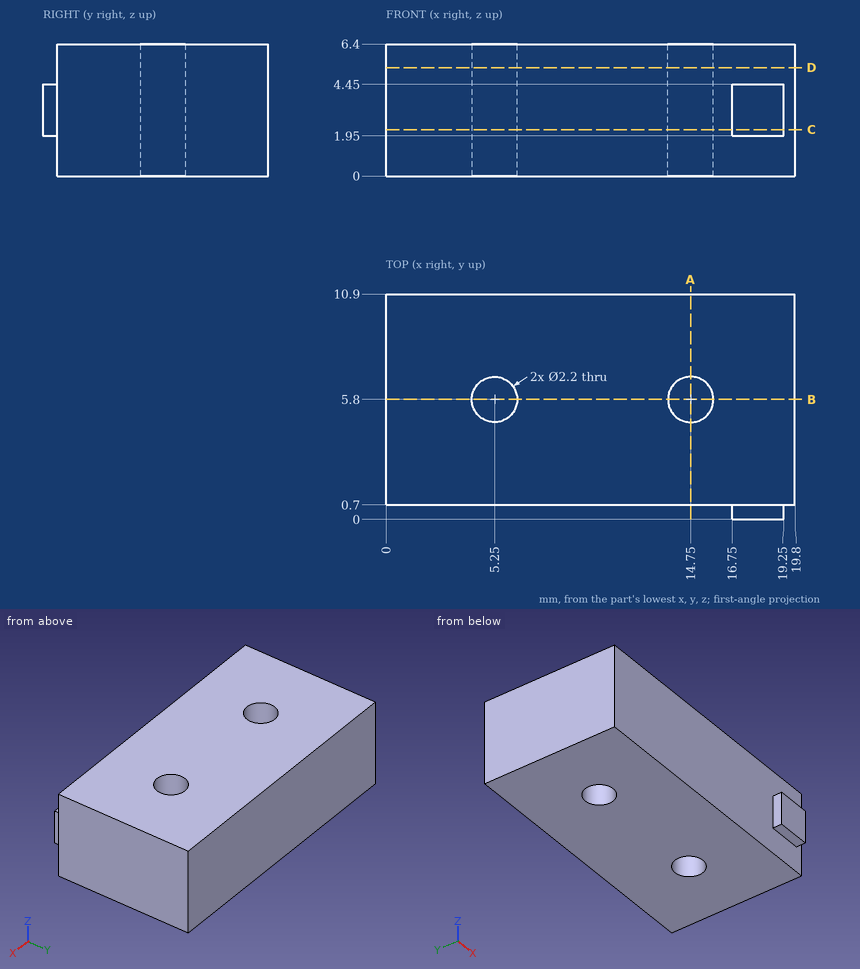
Can you work these out from the drawing? Everything is in mm from the part's minimum corner. Round coordinates to 2 decimals unless told otherwise and drop trailing zeros. Write each loop counter-clockwise with the first axis right and the second up, starting at its lowest first coordinate (ties: lowest second). Pieces come first, ordered by that corner, then holes.
1. Suppose I cut it at D-D (z = 5.25). List the corners of the cut face in (x, y) for me, and give its area (3 significant figures).
2. Suppose I cut it at A-A (x = 14.75). List the corners of the cut face in (y, z) for me.
3. Suppose I cut it at B-B (y = 5.8). List the corners of the cut face in (x, z) for me.
4. I need wall thicknesses on L1, parallel to X at y = 5.8, z = 4; L2, parallel to Y at x = 14.75, z = 2.5; L3, parallel to Y at x = 8.5, z = 1.25. Which ranges of each line are inside material? Lowest first, please.
5. Suppose I cut it at C-C (z = 2.25). List the corners of the cut face in (x, y) for me, and give its area (3 significant figures).
6. Will these pins go through, and if not, where does the flat tip stop? pin 1 Ø0.6 at (y, z) = (0, 3.5) entering from -X; pin 2 Ø1.9 at (x, z) = (11, 3) entering from -Y.
Answer sheet:
1. outline: (0, 0.7) - (19.8, 0.7) - (19.8, 10.9) - (0, 10.9) - close; hole circle Ø2.2 at (5.25, 5.8); hole circle Ø2.2 at (14.75, 5.8)
1. area: 194 mm2
2. outline: (0.7, 0) - (4.7, 0) - (4.7, 6.4) - (0.7, 6.4) - close; (6.9, 0) - (10.9, 0) - (10.9, 6.4) - (6.9, 6.4) - close
3. outline: (0, 0) - (4.15, 0) - (4.15, 6.4) - (0, 6.4) - close; (6.35, 0) - (13.65, 0) - (13.65, 6.4) - (6.35, 6.4) - close; (15.85, 0) - (19.8, 0) - (19.8, 6.4) - (15.85, 6.4) - close
4. L1: x = 0 to 4.15, 6.35 to 13.65, 15.85 to 19.8
4. L2: y = 0.7 to 4.7, 6.9 to 10.9
4. L3: y = 0.7 to 10.9
5. outline: (0, 0.7) - (16.75, 0.7) - (16.75, 0) - (19.25, 0) - (19.25, 0.7) - (19.8, 0.7) - (19.8, 10.9) - (0, 10.9) - close; hole circle Ø2.2 at (5.25, 5.8); hole circle Ø2.2 at (14.75, 5.8)
5. area: 196 mm2
6. pin 1: stops at x = 16.75
6. pin 2: stops at y = 0.7
